Here's how the part is built. I have some questions about the finished solid (model axes, mm). Face numbers are marked on the shaded views. A direction names the side the tool comes from. Coordinates: 2 decimals unless noted, no trailing zeros. Order: outer loops, then holes, each group sorted by start corner. A loop starts at its lowest first (then second) coordinate and runs counter-clockwise, first axis right, second up. Notation, with made-up numbers: (53.5, -1.75) - (95.5, -1.75) arc R18 cw to (95.5, 28.25) - close; hole circle Ø8 at (-11, 31.5). An arc over 180 degrees is marked (long way). Answer in a Markdown table with one row per item. Add a question column.
Item 1: If I drill on line 1 along Y through (x, z) = (-8, 33); line 2 along Y through (x, z) = (-51.5, 41.5); line 3 along X through (y, z) = (-3, 29.5), over which ranges is the centre line in solid material (lowest first)? Write a range as from..to.
Item 2: Will these pins go through, and if not, where does the flat tip stop? pin 1 Ø4.5 at (y, z) = (15.1, 11.8) entering from -X; pin 2 Ø2 at (x, y) = (-46.03, 42.7) entering from -Z; pin 3 Ø2.5 at (x, y) = (40, 44) entering from +Z; pin 4 Ø25 at (y, z) = (-10, 58.5) entering from +X.
Item 3: I want a section at D-D (z = 11.8). Count the separate pieces of the cut face and the enclosed holes in it, plus the area to 3 significant figures.
Item 4: On a 3-axis mill with a long thin cutter (end or side, diameter ignored), from which of +Z, -Z, +X, -X, +Y, -Y can I reach the whole of each face in a straight line? I mean the marked faces 1, 2 and 3. Say none if no direction works.
Item 5: Thinking about a two-plate mould opening in X: for the marked faces 4, 5, 6 and 7, which applies, +X half, -X half, draft (parallel to the pull), parting line (faces both ways), or undercut?
Item 6: I want a section at C-C (x = 22.5). Please give me the cut outline in (y, z).
Item 7: I want a section at A-A (z = 3.5). Please give me the cut outline in (x, y), plus the area to 3 significant figures.
Item 8: I want a section at B-B (y = 0). Please give me the cut outline in (x, z).
```python
from build123d import *
from build123d.topology import SkipClean

# Parameters (mm, degrees)
BOSS_EXTRUDE1_DEPTH = 65
BOSS_EXTRUDE3_START = 3
BOSS_EXTRUDE3_DEPTH = 3
SKETCH4_R           = 19.75
CUT_EXTRUDE1_DEPTH  = 132
SKETCH8_R           = 1.8
BOSS_EXTRUDE6_DEPTH = 60
FILLET1_R           = 7.5
FILLET2_R           = 7.5
FILLET3_R           = 7.5
FILLET4_R           = 7.5
BOSS_EXTRUDE8_DEPTH = 10
FILLET8_R           = 4
CUT_EXTRUDE2_START  = -40
SKETCH13_R          = 1.8
CUT_EXTRUDE2_DEPTH  = 40
SKETCH14_R          = 2.75
CUT_EXTRUDE3_DEPTH  = 3
CUT_EXTRUDE4_DEPTH  = 11.8
SKETCH16_R          = 2.5
CUT_EXTRUDE5_DEPTH  = 12.8
SKETCH18_W          = 9.402156545
SKETCH18_H          = 47.685659657
SKETCH18_W_2        = 10.670772927
CUT_EXTRUDE6_DEPTH  = 23.8


with BuildPart() as part:
    # Sketch1 → Boss-Extrude1 (new body)
    with BuildSketch(Plane(origin=(0, 0, 0), x_dir=(0, 1, 0), z_dir=(0, 0, 1))):
        with BuildLine():
            Line((-49.5, 54.724137931), (-49.5, -54.724137931))
            ThreePointArc((-49.5, -54.724137931), (-47.742640687, -58.966778618), (-43.5, -60.724137931))
            Line((-43.5, -60.724137931), (43.5, -60.724137931))
            ThreePointArc((43.5, -60.724137931), (47.742640687, -58.966778618), (49.5, -54.724137931))
            Line((49.5, -54.724137931), (49.5, 54.724137931))
            ThreePointArc((49.5, 54.724137931), (47.742640687, 58.966778618), (43.5, 60.724137931))
            Line((43.5, 60.724137931), (-43.5, 60.724137931))
            ThreePointArc((-43.5, 60.724137931), (-47.742640687, 58.966778618), (-49.5, 54.724137931))
        make_face()
        with BuildLine():
            Line((-40.5, 57.724137931), (40.5, 57.724137931))
            ThreePointArc((40.5, 57.724137931), (44.742640687, 55.966778618), (46.5, 51.724137931))
            Line((46.5, 51.724137931), (46.5, -51.724137931))
            ThreePointArc((46.5, -51.724137931), (44.742640687, -55.966778618), (40.5, -57.724137931))
            Line((40.5, -57.724137931), (-40.5, -57.724137931))
            ThreePointArc((-40.5, -57.724137931), (-44.742640687, -55.966778618), (-46.5, -51.724137931))
            Line((-46.5, -51.724137931), (-46.5, 51.724137931))
            ThreePointArc((-46.5, 51.724137931), (-44.742640687, 55.966778618), (-40.5, 57.724137931))
        make_face(mode=Mode.SUBTRACT)
    extrude(amount=BOSS_EXTRUDE1_DEPTH)

    # Sketch3 → Boss-Extrude3 (add)
    with BuildSketch(Plane(origin=(0, 0, 0), x_dir=(1, 0, 0), z_dir=(0, 0, -1)).offset(BOSS_EXTRUDE3_START)):
        with BuildLine():
            Line((-54.724137931, 49.5), (54.724137931, 49.5))
            ThreePointArc((54.724137931, 49.5), (58.966778618, 47.742640687), (60.724137931, 43.5))
            Line((60.724137931, 43.5), (60.724137931, -43.5))
            ThreePointArc((60.724137931, -43.5), (58.966778618, -47.742640687), (54.724137931, -49.5))
            Line((54.724137931, -49.5), (-54.724137931, -49.5))
            ThreePointArc((-54.724137931, -49.5), (-58.966778618, -47.742640687), (-60.724137931, -43.5))
            Line((-60.724137931, -43.5), (-60.724137931, 43.5))
            ThreePointArc((-60.724137931, 43.5), (-58.966778618, 47.742640687), (-54.724137931, 49.5))
        make_face()
    extrude(amount=-BOSS_EXTRUDE3_DEPTH)

    # Sketch4 → Cut-Extrude1 (cut)
    with BuildSketch(Plane.YZ.offset(60.724137931)):
        with Locations((0, 65)):
            Circle(SKETCH4_R)
    extrude(amount=-CUT_EXTRUDE1_DEPTH, mode=Mode.SUBTRACT)

    # Sketch8 → Boss-Extrude6 (add)
    # profile 1 of 4: a face of its own
    with BuildSketch(Plane.XY):
        with BuildLine():
            Line((-34.332324886, -38.9), (-57.724137931, -38.9))
            Line((-57.724137931, -38.9), (-57.724137931, -40.5))
            ThreePointArc((-57.724137931, -40.5), (-55.966778618, -44.742640687), (-51.724137931, -46.5))
            Line((-51.724137931, -46.5), (-34.332324886, -46.5))
            Line((-34.332324886, -46.5), (-34.332324886, -38.9))
        make_face()
        with Locations((-46.028231409, -42.7)):
            Circle(SKETCH8_R, mode=Mode.SUBTRACT)
    # profile 2 of 4: a face of its own
    with BuildSketch(Plane.XY):
        with BuildLine():
            Line((-34.332324886, 46.5), (-51.724137931, 46.5))
            ThreePointArc((-51.724137931, 46.5), (-55.966778618, 44.742640687), (-57.724137931, 40.5))
            Line((-57.724137931, 40.5), (-57.724137931, 38.9))
            Line((-57.724137931, 38.9), (-34.332324886, 38.9))
            Line((-34.332324886, 38.9), (-34.332324886, 46.5))
        make_face()
        with Locations((-46.028231409, 42.7)):
            Circle(SKETCH8_R, mode=Mode.SUBTRACT)
    # profile 3 of 4: a face of its own
    with BuildSketch(Plane.XY):
        with BuildLine():
            Line((51.724137931, 46.5), (34.332324886, 46.5))
            Line((34.332324886, 46.5), (34.332324886, 38.9))
            Line((34.332324886, 38.9), (57.724137931, 38.9))
            Line((57.724137931, 38.9), (57.724137931, 40.5))
            ThreePointArc((57.724137931, 40.5), (55.966778618, 44.742640687), (51.724137931, 46.5))
        make_face()
        with Locations((46.028231409, 42.7)):
            Circle(SKETCH8_R, mode=Mode.SUBTRACT)
    # profile 4 of 4: a face of its own
    with BuildSketch(Plane.XY):
        with BuildLine():
            Line((57.724137931, -40.5), (57.724137931, -38.9))
            Line((57.724137931, -38.9), (34.332324886, -38.9))
            Line((34.332324886, -38.9), (34.332324886, -46.5))
            Line((34.332324886, -46.5), (51.724137931, -46.5))
            ThreePointArc((51.724137931, -46.5), (55.966778618, -44.742640687), (57.724137931, -40.5))
        make_face()
        with Locations((46.028231409, -42.7)):
            Circle(SKETCH8_R, mode=Mode.SUBTRACT)
    extrude(amount=BOSS_EXTRUDE6_DEPTH)

    # Fillet1
    fillet1_edges = [part.edges().sort_by_distance(p)[0] for p in [
        (-34.332324886, 46.5, 30),
    ]]
    fillet(fillet1_edges, radius=FILLET1_R)

    # Fillet2
    fillet2_edges = [part.edges().sort_by_distance(p)[0] for p in [
        (34.332324886, 46.5, 30),
    ]]
    fillet(fillet2_edges, radius=FILLET2_R)

    # Fillet3
    fillet3_edges = [part.edges().sort_by_distance(p)[0] for p in [
        (-34.332324886, -46.5, 30),
    ]]
    fillet(fillet3_edges, radius=FILLET3_R)

    # Fillet4
    fillet4_edges = [part.edges().sort_by_distance(p)[0] for p in [
        (34.332324886, -46.5, 30),
    ]]
    fillet(fillet4_edges, radius=FILLET4_R)

    # Sketch12 → Boss-Extrude8 (add, symmetric)
    with SkipClean():  # the faces are left unmerged after this step: merging them gives an invalid solid
        with BuildSketch(Plane(origin=(57.724137931, 0, 0), x_dir=(0, -1, 0), z_dir=(-1, 0, 0))):
            with BuildLine():
                Line((-19.75, 65), (-22.75, 65))
                ThreePointArc((-22.75, 65), (0, 42.25), (22.75, 65))
                Line((22.75, 65), (19.75, 65))
                ThreePointArc((19.75, 65), (0, 45.25), (-19.75, 65))
            make_face()
        boss_extrude8 = extrude(amount=BOSS_EXTRUDE8_DEPTH, both=True)
    add(part.part.scale(1), mode=Mode.REPLACE)  # the faces are merged on a copy

    # Mirror2: Boss-Extrude8 across plane
    add(boss_extrude8.mirror(Plane(origin=(0, 0, 0), x_dir=(0, 0, 1), z_dir=(1, 0, 0))))

    # Fillet8
    fillet8_edges = [part.edges().sort_by_distance(p)[0] for p in [
        (-58.966778618, 47.742640687, -3),
        (0, 49.5, -3),
        (58.966778618, 47.742640687, -3),
        (60.724137931, 0, -3),
        (58.966778618, -47.742640687, -3),
        (0, -49.5, -3),
        (-58.966778618, -47.742640687, -3),
        (-60.724137931, 0, -3),
    ]]
    fillet(fillet8_edges, radius=FILLET8_R)

    # Sketch13 → Cut-Extrude2 (cut)
    with BuildSketch(Plane.XY.offset(CUT_EXTRUDE2_START)):
        with Locations((-46.028231409, 42.7)):
            Circle(SKETCH13_R)
        with Locations((46.028231409, 42.7)):
            Circle(SKETCH13_R)
        with Locations((-46.028231409, -42.7)):
            Circle(SKETCH13_R)
        with Locations((46.028231409, -42.7)):
            Circle(SKETCH13_R)
    extrude(amount=CUT_EXTRUDE2_DEPTH, mode=Mode.SUBTRACT)

    # Sketch14 → Cut-Extrude3 (cut)
    with BuildSketch(Plane(origin=(0, 0, -3), x_dir=(1, 0, 0), z_dir=(0, 0, -1))):
        with Locations(Location((-46.028231409, 42.7, 0), (0, 0, 180))):
            Circle(SKETCH14_R)
        with Locations(Location((-46.028231409, -42.7, 0), (0, 0, 180))):
            Circle(SKETCH14_R)
        with Locations(Location((46.028231409, -42.7, 0), (0, 0, 180))):
            Circle(SKETCH14_R)
        with Locations(Location((46.028231409, 42.7, 0), (0, 0, 180))):
            Circle(SKETCH14_R)
    extrude(amount=-CUT_EXTRUDE3_DEPTH, mode=Mode.SUBTRACT)

    # Sketch15 → Cut-Extrude4 (cut)
    with BuildSketch(Plane(origin=(-60.724137931, 0, 0), x_dir=(0, -1, 0), z_dir=(-1, 0, 0))):
        with BuildLine():
            Line((-34.5, 17.3), (-25.5, 17.3))
            ThreePointArc((-25.5, 17.3), (-24.085786438, 16.714213562), (-23.5, 15.3))
            Line((-23.5, 15.3), (-23.5, 8.3))
            ThreePointArc((-23.5, 8.3), (-24.085786438, 6.885786438), (-25.5, 6.3))
            Line((-25.5, 6.3), (-34.5, 6.3))
            ThreePointArc((-34.5, 6.3), (-35.914213562, 6.885786438), (-36.5, 8.3))
            Line((-36.5, 8.3), (-36.5, 15.3))
            ThreePointArc((-36.5, 15.3), (-35.914213562, 16.714213562), (-34.5, 17.3))
        make_face()
    extrude(amount=-CUT_EXTRUDE4_DEPTH, mode=Mode.SUBTRACT)

    # Sketch16 → Cut-Extrude5 (cut)
    with BuildSketch(Plane(origin=(-60.724137931, 0, 0), x_dir=(0, -1, 0), z_dir=(-1, 0, 0))):
        with Locations(Location((-15.101265496, 11.8, 0), (0, 0, 90))):
            Circle(SKETCH16_R)
    extrude(amount=-CUT_EXTRUDE5_DEPTH, mode=Mode.SUBTRACT)

    # Sketch18 → Cut-Extrude6 (cut)
    with BuildSketch(Plane.XY.offset(65)):
        with Locations((-65.425216203, -1.092829829)):
            Rectangle(SKETCH18_W, SKETCH18_H)
        with Locations((66.059524395, -1.092829829)):
            Rectangle(SKETCH18_W_2, SKETCH18_H)
    extrude(amount=-CUT_EXTRUDE6_DEPTH, mode=Mode.SUBTRACT)


solid = part.part
```
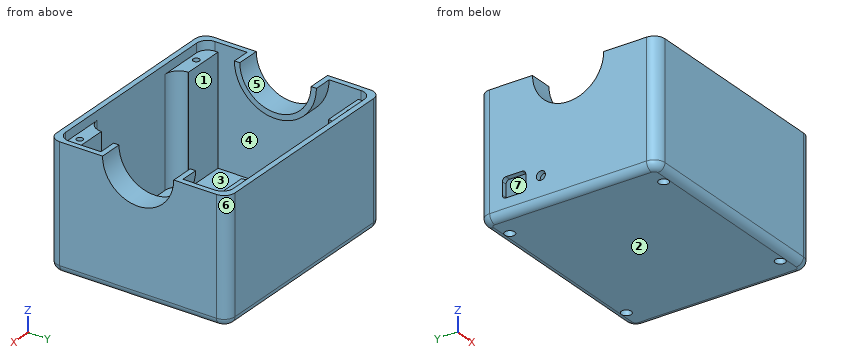
Values follow:
| question | item | result |
|---|---|---|
| 1 | line 1 | y = -49.5..-46.5, 46.5..49.5 |
| 1 | line 2 | y = -49.5..-38.9, 38.9..49.5 |
| 1 | line 3 | x = -60.72..-57.72, 57.72..60.72 |
| 2 | pin 1 | stops at x = 57.72 |
| 2 | pin 2 | passes through |
| 2 | pin 3 | stops at z = 60 |
| 2 | pin 4 | stops at x = 60.72 |
| 3 | separate pieces | 2 |
| 3 | enclosed holes | 4 |
| 3 | area | 1,920 mm^2 |
| 4 | face 1 | +Z |
| 4 | face 2 | -Z, +X, -X, +Y, -Y |
| 4 | face 3 | none |
| 5 | face 4 | undercut |
| 5 | face 5 | draft |
| 5 | face 6 | +X half |
| 5 | face 7 | undercut |
| 6 | outline | (-49.5, 1) arc R4 ccw to (-45.5, -3) - (45.5, -3) arc R4 ccw to (49.5, 1) - (49.5, 65) - (46.5, 65) - (46.5, 0) - (-46.5, 0) - (-46.5, 65) - (-49.5, 65) - close |
| 7 | outline | (-60.72, -43.5) arc R6 ccw to (-54.72, -49.5) - (54.72, -49.5) arc R6 ccw to (60.72, -43.5) - (60.72, 43.5) arc R6 ccw to (54.72, 49.5) - (-54.72, 49.5) arc R6 ccw to (-60.72, 43.5) - close; hole (-57.72, -38.9) - (-34.33, -38.9) - (-34.33, -39) arc R7.5 ccw to (-26.83, -46.5) - (26.83, -46.5) arc R7.5 ccw to (34.33, -39) - (34.33, -38.9) - (57.72, -38.9) - (57.72, 38.9) - (34.33, 38.9) - (34.33, 39) arc R7.5 ccw to (26.83, 46.5) - (-26.83, 46.5) arc R7.5 ccw to (-34.33, 39) - (-34.33, 38.9) - (-57.72, 38.9) - close; hole circle Ø3.6 at (-46.03, -42.7); hole circle Ø3.6 at (-46.03, 42.7); hole circle Ø3.6 at (46.03, -42.7); hole circle Ø3.6 at (46.03, 42.7) |
| 7 | area | 1,970 mm^2 |
| 8 | outline | (-60.72, 1) arc R4 ccw to (-56.72, -3) - (56.72, -3) arc R4 ccw to (60.72, 1) - (60.72, 45.25) - (47.72, 45.25) - (47.72, 42.25) - (57.72, 42.25) - (57.72, 0) - (-57.72, 0) - (-57.72, 42.25) - (-47.72, 42.25) - (-47.72, 45.25) - (-60.72, 45.25) - close |
